Source: CAD feature listing. Evaluate the final solid. Frame: model axes, mm. Face numbers are marked on the shaded views. A direction names the side the tool comes from. Round coordinates to 2 decimals unless told otherwise and drop trailing zeros. Loops run counter-clockwise (first coordinate to the right, second up) from the corner with the lowest first, then second, coordinate; pieces in that order, holes last. Notation, with made-up numbers: (9.5, 8) - (59.5, 8) arc R16 cw to (59.5, 12) - close; hole circle Ø8 at (-0.75, -15.75). An arc over 180 degrees is marked (long way). One line per question, with ' | ' between items. Start each with the question number.
1. Cut plane C-C (y = -14.25). Return loops of the section in (x, z).
2. Cut plane A-A (x = 8.25). State how many separate pieces and enclosed holes the cut face has, then the cut area to 4 significant figures.
3. Cut plane B-B (y = -21.75). Return loops of the section in (x, z).
4. Access query for the marked faces 1, 2 and 3. Directions: +Z, -Z, +X, -X, +Y, -Y. A direction counts if a zero-diameter tool reaches every point of the face in a straight line with its end or side. Return the directions, or none.
5. Ray query, line 1 (Z direction, x = 9, y = -4.25); line 2 (Z direction, x = -16.5, y = -15.5); line 3 (Z direction, x = -10.5, y = -6.5). Return the intervals inside material, ascending.
6. Cut plane D-D (x = -14.5). Return loops of the section in (y, z).
7. Pin query (flat end, axial travel): pin 1 (2.5 mm diameter, centred on x = -9, y = -5.5, fed in from -Z); pin 2 (22 mm diameter, centred on x = 7, z = 11.5, fed in from -Y); pin 3 (5.5 mm diameter, centred on x = 0.5, z = -28, fed in from -Y). Return the tip coordinate at first contact, or that it passes through.
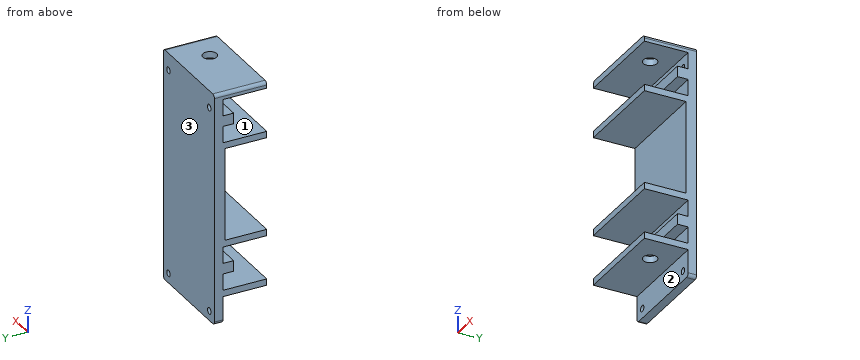
```python
from build123d import *

# Parameters (mm, degrees)
SKETCH1_R           = 1.5
BOSS_EXTRUDE1_DEPTH = 4
SKETCH3_W           = 45
SKETCH3_H           = 3
SKETCH3_H_2         = 5
BOSS_EXTRUDE2_DEPTH = 20.5
SKETCH4_W           = 45
SKETCH4_H           = 5
CUT_EXTRUDE1_DEPTH  = 15.5
SKETCH5_W           = 45
SKETCH5_H           = 43.5
BOSS_EXTRUDE3_DEPTH = 1
SKETCH6_R           = 3.25
CUT_EXTRUDE2_DEPTH  = 103
SKETCH7_W           = 45
SKETCH7_H           = 3
BOSS_EXTRUDE4_DEPTH = 24.5


with BuildPart() as part:
    # Sketch1 → Boss-Extrude1 (new body)
    with BuildSketch(Plane(origin=(0, 0, 0), x_dir=(1, 0, 0), z_dir=(0, 1, 0))):
        with BuildLine():
            Line((21, -54.5), (-21, -54.5))
            ThreePointArc((-21, -54.5), (-22.060660172, -54.060660172), (-22.5, -53))
            Line((-22.5, -53), (-22.5, 53))
            ThreePointArc((-22.5, 53), (-22.060660172, 54.060660172), (-21, 54.5))
            Line((-21, 54.5), (21, 54.5))
            ThreePointArc((21, 54.5), (22.060660172, 54.060660172), (22.5, 53))
            Line((22.5, 53), (22.5, -53))
            ThreePointArc((22.5, -53), (22.060660172, -54.060660172), (21, -54.5))
        make_face()
        with Locations((17.925, -46.425)):
            Circle(SKETCH1_R, mode=Mode.SUBTRACT)
        with Locations((-17.925, -46.425)):
            Circle(SKETCH1_R, mode=Mode.SUBTRACT)
        with Locations((17.925, 49.925)):
            Circle(SKETCH1_R, mode=Mode.SUBTRACT)
        with Locations((-17.925, 49.925)):
            Circle(SKETCH1_R, mode=Mode.SUBTRACT)
    extrude(amount=-BOSS_EXTRUDE1_DEPTH)

    # Sketch3 → Boss-Extrude2 (add)
    with BuildSketch(Plane.XZ.offset(4)):
        with Locations((0, -17)):
            Rectangle(SKETCH3_W, SKETCH3_H)
        with Locations((0, -28.75)):
            Rectangle(SKETCH3_W, SKETCH3_H_2)
        with Locations((0, -40.5)):
            Rectangle(SKETCH3_W, SKETCH3_H)
        with Locations((0, 41.25)):
            Rectangle(SKETCH3_W, SKETCH3_H_2)
        with BuildLine():
            Line((-22.5, 51.5), (22.5, 51.5))
            Line((22.5, 51.5), (22.5, 53))
            ThreePointArc((22.5, 53), (22.060660172, 54.060660172), (21, 54.5))
            Line((21, 54.5), (-21, 54.5))
            ThreePointArc((-21, 54.5), (-22.060660172, 54.060660172), (-22.5, 53))
            Line((-22.5, 53), (-22.5, 51.5))
        make_face()
        with Locations((0, 29.5)):
            Rectangle(SKETCH3_W, SKETCH3_H)
    extrude(amount=BOSS_EXTRUDE2_DEPTH)

    # Sketch4 → Cut-Extrude1 (cut)
    with BuildSketch(Plane.XZ.offset(24.5)):
        with Locations((0, 41.25)):
            Rectangle(SKETCH4_W, SKETCH4_H)
        with Locations((0, -28.75)):
            Rectangle(SKETCH4_W, SKETCH4_H)
    extrude(amount=-CUT_EXTRUDE1_DEPTH, mode=Mode.SUBTRACT)

    # Sketch5 → Boss-Extrude3 (add)
    with BuildSketch(Plane.XZ.offset(4)):
        with Locations((0, 6.25)):
            Rectangle(SKETCH5_W, SKETCH5_H)
    extrude(amount=BOSS_EXTRUDE3_DEPTH)

    # Sketch6 → Cut-Extrude2 (cut)
    with BuildSketch(Plane.XY.offset(54.5)):
        with Locations((8.25, -14.25)):
            Circle(SKETCH6_R)
    extrude(amount=-CUT_EXTRUDE2_DEPTH, mode=Mode.SUBTRACT)

    # Sketch7 → Boss-Extrude4 (add)
    with BuildSketch(Plane.XZ.offset(24.5)):
        with Locations((0, 29.5)):
            Rectangle(SKETCH7_W, SKETCH7_H)
        with Locations((0, -17)):
            Rectangle(SKETCH7_W, SKETCH7_H)
    extrude(amount=-BOSS_EXTRUDE4_DEPTH)


solid = part.part
```
Answers follow:
1) outline: (-22.5, -42) - (5, -42) - (5, -39) - (-22.5, -39) - close; (-22.5, -18.5) - (22.5, -18.5) - (22.5, -15.5) - (-22.5, -15.5) - close; (-22.5, 28) - (22.5, 28) - (22.5, 31) - (-22.5, 31) - close; (-22.5, 51.5) - (5, 51.5) - (5, 54.5) - (-21, 54.5) arc R1.5 ccw to (-22.5, 53) - close; (11.5, -42) - (22.5, -42) - (22.5, -39) - (11.5, -39) - close; (11.5, 51.5) - (22.5, 51.5) - (22.5, 53) arc R1.5 ccw to (21, 54.5) - (11.5, 54.5) - close
2) separate pieces: 3 | enclosed holes: 0 | area: 736.5 mm2
3) outline: (-22.5, -42) - (22.5, -42) - (22.5, -39) - (-22.5, -39) - close; (-22.5, -18.5) - (22.5, -18.5) - (22.5, -15.5) - (-22.5, -15.5) - close; (-22.5, 28) - (22.5, 28) - (22.5, 31) - (-22.5, 31) - close; (-22.5, 51.5) - (22.5, 51.5) - (22.5, 53) arc R1.5 ccw to (21, 54.5) - (-21, 54.5) arc R1.5 ccw to (-22.5, 53) - close
4) face 1: +X, -X, -Y | face 2: -Z, +X, -X, -Y | face 3: +Z, -Z, +X, -X, +Y
5) line 1: z = -42 to -39, -31.25 to -26.25, -18.5 to 31, 38.75 to 43.75, 51.5 to 54.5 | line 2: z = -42 to -39, -18.5 to -15.5, 28 to 31, 51.5 to 54.5 | line 3: z = -42 to -39, -31.25 to -26.25, -18.5 to -15.5, 28 to 31, 38.75 to 43.75, 51.5 to 54.5
6) outline: (-24.5, -42) - (-4, -42) - (-4, -54.5) - (0, -54.5) - (0, 54.5) - (-24.5, 54.5) - (-24.5, 51.5) - (-4, 51.5) - (-4, 43.75) - (-9, 43.75) - (-9, 38.75) - (-4, 38.75) - (-4, 31) - (-24.5, 31) - (-24.5, 28) - (-5, 28) - (-5, -15.5) - (-24.5, -15.5) - (-24.5, -18.5) - (-4, -18.5) - (-4, -26.25) - (-9, -26.25) - (-9, -31.25) - (-4, -31.25) - (-4, -39) - (-24.5, -39) - close
7) pin 1: stops at z = -42 | pin 2: stops at y = -5 | pin 3: stops at y = -9
